Input: part model. Units: mm. Frame: model coordinates. A direction names the side the tool comes from. Coordinates: 2 decimals unless noted, no trailing zeros. Loops run counter-clockwise (first coordinate to the right, second up) from the corner with the lowest first, then second, coordinate; pieces in that order, holes last. Notation, with made-up numbers: (63.25, 58.25) - (108.25, 58.25) arc R25 ccw to (108.25, 92.25) - close; hole circle Ø1 at (70.5, 29). An arc over 180 degrees is marked (long way). Use one line per item in the form item = value.
from build123d import *

# Parameters (mm, degrees)
SKETCH1_W           = 9.72
SKETCH1_H           = 20
SKETCH1_R           = 1.5
BOSS_EXTRUDE1_DEPTH = 2
BOSS_EXTRUDE2_DEPTH = 20
SKETCH3_R           = 0.75
BOSS_EXTRUDE3_DEPTH = 1.53


with BuildPart() as part:
    # Sketch1 → Boss-Extrude1 (new body)
    with BuildSketch(Plane.XY):
        with Locations((4.86, 10)):
            Rectangle(SKETCH1_W, SKETCH1_H)
        with Locations((2.72, 16)):
            Circle(SKETCH1_R, mode=Mode.SUBTRACT)
        with Locations((2.72, 4)):
            Circle(SKETCH1_R, mode=Mode.SUBTRACT)
    extrude(amount=BOSS_EXTRUDE1_DEPTH)

    # Sketch2 → Boss-Extrude2 (add)
    with BuildSketch(Plane.XZ):
        with BuildLine():
            Line((9.72, 2), (9.72, 0))
            ThreePointArc((9.72, 0), (11.367131495, 0.954473399), (11.999702326, 2.75))
            Line((11.999702326, 2.75), (10.47, 2.75))
            ThreePointArc((10.47, 2.75), (10.250330086, 2.219669914), (9.72, 2))
        make_face()
    extrude(amount=-BOSS_EXTRUDE2_DEPTH)

    # Sketch3 → Boss-Extrude3 (add)
    with BuildSketch(Plane(origin=(12, 0, 0), x_dir=(0, 0, -1), z_dir=(1, 0, 0))):
        with BuildLine():
            Line((-2.75, 20), (-5, 20))
            ThreePointArc((-5, 20), (-7.121320344, 19.121320344), (-8, 17))
            Line((-8, 17), (-8, 3))
            ThreePointArc((-8, 3), (-7.121320344, 0.878679656), (-5, 0))
            Line((-5, 0), (-2.75, 0))
            Line((-2.75, 0), (-2.75, 20))
        make_face()
        with Locations((-6, 10)):
            Circle(SKETCH3_R, mode=Mode.SUBTRACT)
    extrude(amount=-BOSS_EXTRUDE3_DEPTH)


solid = part.part
Q1. Pull-direction query (X, two-part tool) for faces 3 (the flat face through (12, 10, 5)), 4 (the cylindrical face through (1.6, 17, 1)), 5 (the flat face through (5, 10, 2)), 6 (the cylindrical face through (1.6, 5, 1)); classes: pulls with the +X half, pulls with the -X half, needs draft (parallel to the pull), parting line crosses it, or undercut.
Check values:
face_3 = pulls with the +X half
face_4 = undercut
face_5 = needs draft
face_6 = undercut
Q2. Set-up query: faces 1 (the flat face through (6, 20, 1)), 2 (the flat face through (10.47, 10, 5)). Return all of +Z, -Z, +X, -X, +Y, -Y with unobstructed straight access to the full face (end or side cutting, diameter ignored); none if empty.
Check values:
face_1 = +Z, -Z, +X, -X, +Y
face_2 = +Z, -X, +Y, -Y
Q3. Cut plane C-C, the plane z = 6. Return loops of the section in (x, y), then the cut area to 3 significant figures.
Check values:
outline = (10.47, 0.17) - (12, 0.17) - (12, 9.25) - (10.47, 9.25) - close; (10.47, 10.75) - (12, 10.75) - (12, 19.83) - (10.47, 19.83) - close
area = 27.8 mm²
Q4. Ray query, line 1 along Y through (x, z) = (2.72, 0.9); line 2 along X through (y, z) = (1.25, 3.75); line 3 along Z through (x, y) = (1.75, 11.5). Return the intervals inside material, ascending. Write a range as [from, to].
Check values:
line_1 = [0, 2.5], [5.5, 14.5], [17.5, 20]
line_2 = [10.47, 12]
line_3 = [0, 2]
Q5. Cut plane B-B, the plane x = 2.72. Return loops of the section in (y, z).
Check values:
outline = (0, 0) - (2.5, 0) - (2.5, 2) - (0, 2) - close; (5.5, 0) - (14.5, 0) - (14.5, 2) - (5.5, 2) - close; (17.5, 0) - (20, 0) - (20, 2) - (17.5, 2) - close
Q6. First-contact query: P1, Ø1.5, axis at x = 10.5, y = 3, coming from the -Z side; P2, Ø2.5, axis at y = 13.5, z = 5.5, coming from the -X side. Flat tips, straight axial feed; report the tip coordinate or a pass-through.
Check values:
P1 = 0.01
P2 = 10.47
